Part model, mm, in its own coordinate system. A direction names the side the tool comes from. Coordinates: 2 decimals unless noted, no trailing zeros. Order: outer loops, then holes, each group sorted by start corner. A loop starts at its lowest first (then second) coordinate and runs counter-clockwise, first axis right, second up.
1) Cut at A-A (z = 4.8). List the corners of the cut face in (x, y).
2) Pin check, flat tips, straight feed: pin 1 Ø11 at (x, y) = (1.5, 11) entering from +Z; pin 2 Ø3 at (y, z) = (0.5, 1) entering from -X; pin 3 Ø1.2 at (x, z) = (-3, 3) entering from +Y; pin 4 Ø1.8 at (x, y) = (-10.05, 23.5) entering from -Z. Stop position of each tip, or through.
3) Mould opens along X. For faces 1 (the flat face through (-15, 27, 6)), 2 (the cylindrical face through (-15.456, 15.869, 1.972)), 3 (the cylindrical face through (-9.247, 24.765, 3.042)) say: +X half, -X half, draft (parallel to the pull), parting line (faces both ways), or undercut.
4) Cut at B-B (x = 8.5). List the corners of the cut face in (y, z), and give its area (3 significant figures).
5) Wall check: L1, parallel to Y at x = -8, z = 3.2; L2, parallel to Y at x = 3.5, z = 2.3; L3, parallel to X at y = -6.5, z = 3.6. Give the ranges that are in metal, low to high.
6) Tool access for faces 4 (the cylindrical face through (-3.797, -10.359, 1.972)), 5 (the cylindrical face through (10.547, -15.359, 1.972)), 6 (the cylindrical face through (-4.64, 1.817, 2.986)): list every direction of +Z, -Z, +X, -X, +Y, -Y with a clear straight run to the whole face (end or side of a thin tool).
7) Cut at D-D (y = 11). List the corners of the cut face in (x, z).
8) Cut at C-C (y = -9.5). List the corners of the cut face in (x, z).
```python
from build123d import *
from build123d.topology import SkipClean

# Parameters (mm, degrees)
SKETCH_1_R          = 10
SKETCH_1_W          = 23.5
SKETCH_1_H          = 33
SKETCH_1_R_2        = 1.25
EXTRUDE_1_DEPTH     = 4
SKETCH_2_R          = 10
EXTRUDE_2_DEPTH     = 2
SKETCH_3_R          = 1.5
CUT_EXTRUDE_1_DEPTH = 6
SKETCH_4_W          = 10
SKETCH_4_H          = 12
CUT_EXTRUDE_2_DEPTH = 6
CUT_EXTRUDE_START   = -10
CUT_EXTRUDE_4_DEPTH = 10
EXTRUDE_4_DEPTH     = 4
FILLET_1_R          = 4
CUT_EXTRUDE_5_DEPTH = 2
FILLET_2_R          = 2
FILLET_3_R          = 4


with BuildPart() as part:
    # 草图1 → 凸台-拉伸1 (new body)
    # profile 1 of 3: a face of its own
    with BuildSketch(Plane.XY):
        with Locations((-15.25, 26.5)):
            Circle(SKETCH_1_R)
    # profile 2 of 3: a face of its own
    with BuildSketch(Plane.XY):
        with BuildLine():
            Line((-15.25, 16.5), (-11.75, 16.5))
            Line((-11.75, 16.5), (11.75, 16.5))
            Line((11.75, 16.5), (-8.736127865, 34.087454765))
            ThreePointArc((-8.736127865, 34.087454765), (-6.16323156, 30.675001716), (-5.25, 26.5))
            ThreePointArc((-5.25, 26.5), (-8.178932188, 19.428932188), (-15.25, 16.5))
        make_face()
    # profile 3 of 3: a face of its own
    with BuildSketch(Plane.XY):
        Rectangle(SKETCH_1_W, SKETCH_1_H)
        with Locations((-8, -1.5)):
            Circle(SKETCH_1_R_2, mode=Mode.SUBTRACT)
        with Locations((-8, -9.5)):
            Circle(SKETCH_1_R_2, mode=Mode.SUBTRACT)
        with Locations((8, -9.5)):
            Circle(SKETCH_1_R_2, mode=Mode.SUBTRACT)
        with Locations((8, -1.5)):
            Circle(SKETCH_1_R_2, mode=Mode.SUBTRACT)
    extrude(amount=EXTRUDE_1_DEPTH)

    # 草图2 → 凸台-拉伸2 (add)
    with BuildSketch(Plane.XY.offset(4)):
        with Locations(Location((-15.25, 26.5, 0), (0, 0, 270))):
            Circle(SKETCH_2_R)
    extrude(amount=EXTRUDE_2_DEPTH)

    # 草图3 → 切除-拉伸1 (cut)
    with BuildSketch(Plane.XY.offset(6)):
        with Locations((-15.25, 32.5)):
            Circle(SKETCH_3_R)
        with Locations((-10.053847577, 29.5)):
            Circle(SKETCH_3_R)
        with Locations((-10.053847577, 23.5)):
            Circle(SKETCH_3_R)
        with Locations((-15.25, 20.5)):
            Circle(SKETCH_3_R)
        with Locations((-20.446152423, 23.5)):
            Circle(SKETCH_3_R)
        with Locations((-20.446152423, 29.5)):
            Circle(SKETCH_3_R)
    extrude(amount=-CUT_EXTRUDE_1_DEPTH, mode=Mode.SUBTRACT)

    # 草图4 → 切除-拉伸2 (cut)
    with BuildSketch(Plane.XY.offset(4)):
        with Locations((0, -5.5)):
            Rectangle(SKETCH_4_W, SKETCH_4_H)
    extrude(amount=-CUT_EXTRUDE_2_DEPTH, mode=Mode.SUBTRACT)

    # 草图7 → 切除-拉伸4 (cut)
    with SkipClean():  # the faces are left unmerged after this step: merging them gives an invalid solid
        with BuildSketch(Plane.XY.offset(4).offset(CUT_EXTRUDE_START)):
            with BuildLine():
                Line((-7.408855029, 32.706161901), (11.75, 8.5))
                Line((11.75, 8.5), (11.75, 16.5))
                Line((11.75, 16.5), (-8.736127865, 34.087454765))
                ThreePointArc((-8.736127865, 34.087454765), (-8.03933973, 33.428663542), (-7.408855029, 32.706161901))
            make_face()
        extrude(amount=CUT_EXTRUDE_4_DEPTH, mode=Mode.SUBTRACT)

    # 草图8 → 凸台-拉伸4 (add)
    with SkipClean():  # the faces are left unmerged after this step: merging them gives an invalid solid
        with BuildSketch(Plane.XY.offset(4)):
            Polygon((-15.25, 16.5), (-11.75, 8.5), (-11.75, 16.5), align=None)
        extrude(amount=-EXTRUDE_4_DEPTH)

    # 圆角1
    # the kernel refuses this fillet: 4 mm, written as the material it adds along each edge
    with BuildSketch(Plane(origin=(-11.75, 8.5, 4), x_dir=(-0.4008188340197085, 0.9161573349021888, 0), z_dir=(0, 0, -1))) as fillet_1_piece_1:
        with BuildLine():
            CenterArc((FILLET_1_R * 0.209178456653, -FILLET_1_R), FILLET_1_R, 90, 23.629377731)
            Line((-FILLET_1_R * 0.191640377366, -FILLET_1_R * 0.0838426650978), (0, 0))
            Line((0, 0), (FILLET_1_R * 0.209178456653, 0))
        make_face()
    extrude(amount=4)
    with BuildSketch(Plane(origin=(-15.25, 16.5, 0), x_dir=(-0.9951749946983144, 0.09811590048106404, 0), z_dir=(0, 0, 1))) as fillet_1_piece_2:
        with BuildLine():
            CenterArc((2.354781612, 3.980699979), FILLET_1_R, 209.260063678, 55.109250376)
            Line((-1.134859069, 2.025602047), (0, 0))
            ThreePointArc((0, 0), (0.981159005, 0.048250053), (1.96231801, 0))
        make_face()
    extrude(amount=4)
    # the kernel refuses this fillet: 4 mm, written as the material it takes off along each edge
    with BuildSketch(Plane(origin=(11.75, -16.5, -10), x_dir=(0, 1, 0), z_dir=(0, 0, 1)), Plane(origin=(-11.75, -16.5, -10), x_dir=(1, 0, 0), z_dir=(0, 0, 1))) as fillet_1_2_piece_1:
        with BuildLine():
            CenterArc((FILLET_1_R, FILLET_1_R), FILLET_1_R, 180, 90)
            Line((0, FILLET_1_R), (0, 0))
            Line((0, 0), (FILLET_1_R, 0))
        make_face()
    extrude(amount=24, mode=Mode.SUBTRACT)
    with BuildSketch(Plane(origin=(11.75, 8.5, -3.478567049), x_dir=(-0.6206161901076825, 0.7841144971088245, 0), z_dir=(0, 0, 1))) as fillet_1_2_piece_2:
        with BuildLine():
            CenterArc((FILLET_1_R * 0.347856704888, FILLET_1_R), FILLET_1_R, 231.638854085, 38.361145915)
            Line((-FILLET_1_R * 0.272759485219, FILLET_1_R * 0.215885502891), (0, 0))
            Line((0, 0), (FILLET_1_R * 0.347856704888, 0))
        make_face()
    extrude(amount=10.957134098, mode=Mode.SUBTRACT)

    # 草图9 → 切除-拉伸5 (cut)
    with BuildSketch(Plane.XY.offset(4)):
        Polygon((-7.627398855, 7.809036267), (-4.867195488, 1.5), (8.671465121, 1.5), align=None)
        Polygon((-7.160168155, 10.845088414), (10.991392982, 3.818901946), (0.414449212, 17.182289942), align=None)
    extrude(amount=-CUT_EXTRUDE_5_DEPTH, mode=Mode.SUBTRACT)

    # 圆角2
    fillet_2_edges = [part.edges().sort_by_distance(p)[0] for p in [
        (-7.160168155, 10.845088414, 3),
        (0.414449212, 17.182289942, 3),
        (10.991392982, 3.818901946, 3),
        (8.671465121, 1.5, 3),
        (-4.867195488, 1.5, 3),
        (-7.627398855, 7.809036267, 3),
    ]]
    fillet(fillet_2_edges, radius=FILLET_2_R)

    # 圆角3
    fillet_3_edges = [part.edges().sort_by_distance(p)[0] for p in [
        (5, 0.5, 2),
        (5, -11.5, 2),
        (-5, -11.5, 2),
        (-5, 0.5, 2),
    ]]
    fillet(fillet_3_edges, radius=FILLET_3_R)


solid = part.part
```
Geometry check:
1. outline: circle Ø20 at (-15.25, 26.5); hole circle Ø3 at (-20.45, 23.5); hole circle Ø3 at (-20.45, 29.5); hole circle Ø3 at (-15.25, 20.5); hole circle Ø3 at (-15.25, 32.5); hole circle Ø3 at (-10.05, 23.5); hole circle Ø3 at (-10.05, 29.5)
2. pin 1: stops at z = 4
2. pin 2: stops at x = -11.75
2. pin 3: stops at y = 27.89
2. pin 4: passes through
3. face 1: draft
3. face 2: -X half
3. face 3: undercut
4. outline: (-16.43, 0) - (-10.65, 0) - (-10.65, 4) - (-16.43, 4) - close; (-8.35, 0) - (-2.65, 0) - (-2.65, 4) - (-8.35, 4) - close; (-0.35, 0) - (12.61, 0) - (12.61, 4) - (-0.35, 4) - close
4. area: 97.8 mm2
5. L1: y = -16.49 to -10.75, -8.25 to -2.75, -0.25 to 33.39
5. L2: y = -16.5 to -10.62, -0.38 to 6.72, 13.28 to 18.92
5. L3: x = -11.75 to -5, 5 to 11.75
6. face 4: +Z, -Z
6. face 5: +Z, -Z, +X, -Y
6. face 6: +Z
7. outline: (-12.84, 0) - (9.77, 0) - (9.77, 4) - (5.31, 4) - (5.31, 2) - (-5.22, 2) - (-5.22, 4) - (-12.84, 4) - close
8. outline: (-11.75, 0) - (-9.25, 0) - (-9.25, 4) - (-11.75, 4) - close; (-6.75, 0) - (-4.46, 0) - (-4.46, 4) - (-6.75, 4) - close; (4.46, 0) - (6.75, 0) - (6.75, 4) - (4.46, 4) - close; (9.25, 0) - (11.75, 0) - (11.75, 4) - (9.25, 4) - close
